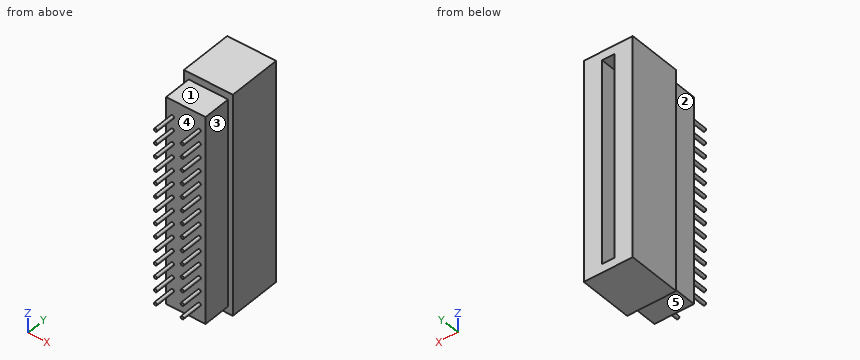
from build123d import *

# Parameters (mm, degrees)
SKETCH001_W           = 9.26
SKETCH001_H           = 10.18
EXTRUDE001_DEPTH      = 1.355
EXTRUDE001_DEPTH_BACK = 0.3
SKETCH002_W           = 9.26
SKETCH002_H           = 10.18
EXTRUDE002_DEPTH      = 1.35
EXTRUDE002_DEPTH_BACK = 0.3
SKETCH003_R           = 0.3
EXTRUDE003_DEPTH      = 4
EXTRUDE_DEPTH         = 39.3


with BuildPart() as extrude001:
    # Sketch001 (on Face14 of Extrude) → Extrude001 (new body, two sides)
    with BuildSketch(Plane.XY.offset(39.3)) as extrude001_sk:
        with Locations((0, 10.39)):
            Rectangle(SKETCH001_W, SKETCH001_H)
    extrude(amount=EXTRUDE001_DEPTH)
    extrude(extrude001_sk.sketch, amount=-EXTRUDE001_DEPTH_BACK)


with BuildPart() as extrude002:
    # Sketch002 (on Face13 of Extrude) → Extrude002 (new body, two sides)
    with BuildSketch(Plane(origin=(0, 0, 0), x_dir=(1, 0, 0), z_dir=(0, 0, -1))) as extrude002_sk:
        with Locations((0, -10.39)):
            Rectangle(SKETCH002_W, SKETCH002_H)
    extrude(amount=EXTRUDE002_DEPTH)
    extrude(extrude002_sk.sketch, amount=-EXTRUDE002_DEPTH_BACK)


with BuildPart() as extrude003:
    # Sketch003 (on Face4 of Extrude) → Extrude003 (new body)
    with BuildSketch(Plane.XZ):
        with Locations((-2.54, 36.16)):
            Circle(SKETCH003_R)
        with Locations((-2.54, 33.62)):
            Circle(SKETCH003_R)
        with Locations((-2.54, 31.08)):
            Circle(SKETCH003_R)
        with Locations((-2.54, 28.54)):
            Circle(SKETCH003_R)
        with Locations((-2.54, 26)):
            Circle(SKETCH003_R)
        with Locations((-2.54, 23.46)):
            Circle(SKETCH003_R)
        with Locations((-2.54, 20.92)):
            Circle(SKETCH003_R)
        with Locations((-2.54, 18.38)):
            Circle(SKETCH003_R)
        with Locations((-2.54, 15.84)):
            Circle(SKETCH003_R)
        with Locations((-2.54, 13.3)):
            Circle(SKETCH003_R)
        with Locations((-2.54, 10.76)):
            Circle(SKETCH003_R)
        with Locations((-2.54, 8.22)):
            Circle(SKETCH003_R)
        with Locations((-2.54, 5.68)):
            Circle(SKETCH003_R)
        with Locations((-2.54, 3.14)):
            Circle(SKETCH003_R)
        with Locations((2.54, 3.14)):
            Circle(SKETCH003_R)
        with Locations((2.54, 5.68)):
            Circle(SKETCH003_R)
        with Locations((2.54, 8.22)):
            Circle(SKETCH003_R)
        with Locations((2.54, 10.76)):
            Circle(SKETCH003_R)
        with Locations((2.54, 13.3)):
            Circle(SKETCH003_R)
        with Locations((2.54, 15.84)):
            Circle(SKETCH003_R)
        with Locations((2.54, 18.38)):
            Circle(SKETCH003_R)
        with Locations((2.54, 20.92)):
            Circle(SKETCH003_R)
        with Locations((2.54, 23.46)):
            Circle(SKETCH003_R)
        with Locations((2.54, 26)):
            Circle(SKETCH003_R)
        with Locations((2.54, 28.54)):
            Circle(SKETCH003_R)
        with Locations((2.54, 31.08)):
            Circle(SKETCH003_R)
        with Locations((2.54, 33.62)):
            Circle(SKETCH003_R)
        with Locations((2.54, 36.16)):
            Circle(SKETCH003_R)
    extrude(amount=EXTRUDE003_DEPTH)


with BuildPart() as fusion:
    # Sketch → Extrude (new body)
    with BuildSketch(Plane.XY):
        Polygon((-4.63, 15.48), (-4.63, 5.3), (-3.735, 5.3), (-3.735, 0), (3.735, 0), (3.735, 5.3), (4.63, 5.3), (4.63, 15.48), (1.17, 15.48), (1.17, 8.6), (-1.17, 8.6), (-1.17, 15.48), align=None)
    extrude(amount=EXTRUDE_DEPTH)

    # Fusion: union Extrude001, Extrude002, Extrude003
    add(extrude001.part)
    add(extrude002.part)
    add(extrude003.part)


solid = fusion.part
The listing builds one solid part. Answer for the finished solid, in the listing's coordinates (mm). Face numbers are marked on the shaded views. A direction names the side the tool comes from. Give positions to 0.01 mm unless a question says otherwise; leave off trailing zeros. Write each loop counter-clockwise with the first axis right and the second up, starting at its lowest first coordinate (ties: lowest second). Pieces come first, ordered by that corner, then holes.
1) Section B-B (z = 9) is taken. Write down the section's boundary in (x, y) (3 decimals).
2) Section D-D (y = 2.75) is taken. Write down the section's boundary in (x, z) (3 decimals), and give its area (3 significant figures).
3) Section C-C (x = 0.25) is taken. Write down the section's boundary in (y, z) (3 decimals).
4) Section A-A (y = 12.5) is taken. Write down the section's boundary in (x, z) (3 decimals), and give its area (3 significant figures).
5) Given P1, Ø4, axis at x = 2, y = 3, coming from the +Z side; P2, Ø3, axis at y = 0.5, z = 29, coming from the -X side (3 decimals); P3, Ø0.7, axis at x = 0, z = 13, coming from the +Y side, each flat-ended and moving along its own axis, determine where each tip first touches the part or whether it passes through.
6) Find the intervals of material crossed by L1, parallel to X at y = 9.25, z = 12.5; L2, parallel to Z at x = 0.5, y = 9.25 (3 decimals); L3, parallel to X at y = -2.75, z = 28.5, in increasing order.
7) A tool of negligible diameter and unlimited length cuts with its end or side. For the marked faces 1, 2, 3, 4 and 5, from which of +Z, -Z, +X, -X, +Y, -Y can it reach the whole face along a straight path? Write none if from no direction.
Response:
1. outline: (-4.63, 5.3) - (-3.735, 5.3) - (-3.735, 0) - (3.735, 0) - (3.735, 5.3) - (4.63, 5.3) - (4.63, 15.48) - (1.17, 15.48) - (1.17, 8.6) - (-1.17, 8.6) - (-1.17, 15.48) - (-4.63, 15.48) - close
2. outline: (-3.735, 0) - (3.735, 0) - (3.735, 39.3) - (-3.735, 39.3) - close
2. area: 294 mm2
3. outline: (0, 0) - (5.3, 0) - (5.3, -1.35) - (15.48, -1.35) - (15.48, 0.3) - (8.6, 0.3) - (8.6, 39) - (15.48, 39) - (15.48, 40.655) - (5.3, 40.655) - (5.3, 39.3) - (0, 39.3) - close
4. outline: (-4.63, -1.35) - (4.63, -1.35) - (4.63, 40.655) - (-4.63, 40.655) - close; hole (-1.17, 0.3) - (1.17, 0.3) - (1.17, 39) - (-1.17, 39) - close
4. area: 298 mm2
5. P1: stops at z = 39.3
5. P2: stops at x = -3.735
5. P3: stops at y = 8.6
6. L1: x = -4.63 to -1.17, 1.17 to 4.63
6. L2: z = -1.35 to 0.3, 39 to 40.655
6. L3: x = -2.84 to -2.24, 2.24 to 2.84
7. face 1: +Z, +X, -X, -Y
7. face 2: +Z, -Z, -X, -Y
7. face 3: +Z, -Z, +X, -Y
7. face 4: -Y
7. face 5: -Z, +X, -X, -Y
